from build123d import *

# Parameters (mm, degrees)
BOSS_EXTRUDE1_DEPTH = 50.8
SKETCH2_W           = 3.175
SKETCH2_H           = 12.446
SKETCH2_R           = 3.175
CUT_EXTRUDE1_DEPTH  = 56.811406764


with BuildPart() as part:
    # Sketch1 → Boss-Extrude1 (new body)
    with BuildSketch(Plane.XY):
        with BuildLine():
            Line((0, 0), (19.05, 0))
            ThreePointArc((19.05, 0), (20.6375, 5.924630657), (16.300369343, 1.5875))
            Line((16.300369343, 1.5875), (17.532203877, 2.2987))
            ThreePointArc((17.532203877, 2.2987), (19.9263, 4.692796123), (19.05, 1.4224))
            Line((19.05, 1.4224), (0, 1.4224))
            Line((0, 1.4224), (0, 0))
        make_face()
    extrude(amount=BOSS_EXTRUDE1_DEPTH)

    # Sketch2 → Cut-Extrude1 (cut, through all)
    with BuildSketch(Plane.XZ):
        with Locations((20.6375, 14.859)):
            Rectangle(SKETCH2_W, SKETCH2_H)
        with Locations((17.4625, 14.859)):
            Rectangle(SKETCH2_W, SKETCH2_H)
        with Locations((20.6375, 35.941)):
            Rectangle(SKETCH2_W, SKETCH2_H)
        with Locations((17.4625, 35.941)):
            Rectangle(SKETCH2_W, SKETCH2_H)
        with Locations(Location((6.985, 43.815, 0), (0, 0, 270))):
            Circle(SKETCH2_R)
        with Locations(Location((6.985, 6.985, 0), (0, 0, 270))):
            Circle(SKETCH2_R)
    extrude(amount=-CUT_EXTRUDE1_DEPTH, mode=Mode.SUBTRACT)


solid = part.part
Check sheet for the modelled part. Datum: model origin and axes. Units: mm. A direction names the side the tool comes from. Give positions to 0.01 mm unless a question says otherwise; leave off trailing zeros. Write each loop counter-clockwise with the first axis right and the second up, starting at its lowest first coordinate (ties: lowest second). Pieces come first, ordered by that corner, then holes. Notation, with made-up numbers: (23, -12) -> (69, -12) arc R19 ccw to (69, 5) -> close; hole circle Ø3 at (-8, -33). An arc over 180 degrees is marked (long way). Use one line per item in the form item = value. Start each with the question number.
1. Section check B-B (x = 9.25). Record the cut outline in (y, z).
2. Section check D-D (y = 0.5). Record the cut outline in (x, z) (3 decimals), and give its area (3 significant figures).
3. Thickness scan on line 1 along Z through (x, y) = (17.25, 5.5); line 2 along Z through (x, y) = (6.25, 0.75); line 3 along Y through (x, z) = (19, 48). Record the ranges inside material, lowest first. Write a range as from..to.
4. Section check A-A (y = 2.75). Record the cut outline in (x, z).
5. Go/stop test with flat-tipped pins: P1, Ø1.5, axis at x = 11, z = 38.5, coming from the +Y side; P2, Ø3, axis at x = 19.05, y = 3.175, coming from the -Z side; P3, Ø1.6, axis at y = 0.5, z = 35.5, coming from the +X side (3 decimals); P4, Ø3, axis at y = 0.5, z = 7.5, coming from the +X side. Record where each tip stops, or that it passes through.
6. Access from +Z, -Z, +X, -X, +Y, -Y to the whole of each face (thin tool, end or side, straight path). Record for faces 1 (the flat face through (16.91, 1.94, 4.26)), 2 (the flat face through (10, 1.422, 25)), 3 (the flat face through (20.4, 1.7, 8.636)).
7. Mould release check, pull along Z, two halves, no side actions. Record for faces 4 (the flat face through (18, 5, 21.082)), 5 (the flat face through (14, 1, 50.8)), 6 (the flat face through (16.91, 1.94, 25.34)), 7 (the flat face through (20.4, 1.7, 29.718)): pulls with the +Z half, pulls with the -Z half, needs draft (parallel to the pull), parting line crosses it, or undercut.
Conclusion:
q1.outline = (0, 0) -> (1.42, 0) -> (1.42, 4.76) -> (0, 4.76) -> close; (0, 9.21) -> (1.42, 9.21) -> (1.42, 41.59) -> (0, 41.59) -> close; (0, 46.04) -> (1.42, 46.04) -> (1.42, 50.8) -> (0, 50.8) -> close
q2.outline = (0, 0) -> (20.76, 0) -> (20.76, 8.636) -> (15.875, 8.636) -> (15.875, 21.082) -> (20.76, 21.082) -> (20.76, 29.718) -> (15.875, 29.718) -> (15.875, 42.164) -> (20.76, 42.164) -> (20.76, 50.8) -> (0, 50.8) -> close; hole circle Ø6.35 at (6.985, 6.985); hole circle Ø6.35 at (6.985, 43.815)
q2.area = 870 mm²
q3.line_1 = 0..8.64, 21.08..29.72, 42.16..50.8
q3.line_2 = 0..3.9, 10.07..40.73, 46.9..50.8
q3.line_3 = 0..1.42, 4.93..6.35
q4.outline = (15.9, 0) -> (17.35, 0) -> (17.35, 8.64) -> (15.9, 8.64) -> close; (15.9, 21.08) -> (17.35, 21.08) -> (17.35, 29.72) -> (15.9, 29.72) -> close; (15.9, 42.16) -> (17.35, 42.16) -> (17.35, 50.8) -> (15.9, 50.8) -> close; (20.75, 0) -> (22.2, 0) -> (22.2, 8.64) -> (20.75, 8.64) -> close; (20.75, 21.08) -> (22.2, 21.08) -> (22.2, 29.72) -> (20.75, 29.72) -> close; (20.75, 42.16) -> (22.2, 42.16) -> (22.2, 50.8) -> (20.75, 50.8) -> close
q5.P1 = 1.42
q5.P2 = through
q5.P3 = 15.875
q5.P4 = 22
q6.face_1 = +Z, -Z
q6.face_2 = +Z, -Z, -X
q6.face_3 = +X, +Y, -Y
q7.face_4 = undercut
q7.face_5 = pulls with the +Z half
q7.face_6 = needs draft
q7.face_7 = undercut
